Here's the drawing with two shaded views (mm, measured from the low corner). I have some questions. A direction names the side the tool comes from. Give positions to 0.01 mm unless a question says otherwise; leave off trailing zeros. Loops run counter-clockwise (first coordinate to the right, second up) from the corner with the lowest first, then second, coordinate; pieces in that order, holes last. Notation, with made-up numbers: (-11, -12) - (44, -12) arc R35 cw to (44, 23) - close; hole circle Ø3 at (57, 86). An arc over 180 degrees is marked (long way). Write each question's results on one line, items separated by ' | '. Start each with the question number.
1) I want a section at C-C, the plane z = 9. Write out the boundary of the cut face in (x, y).
2) I want a section at A-A, the plane y = 30. Write out the boundary of the cut face in (x, z), and give its area (3 significant figures).
3) I want a section at B-B, the plane x = 22.5. Write out the boundary of the cut face in (y, z), and give its area (3 significant figures).
4) I'm going to push flat-ended pins straight in: pin 1 (3 mm diameter, centred on x = 10.5, z = 27.5, fed in from +Y); pin 2 (10 mm diameter, centred on y = 20, z = 8, fed in from +X); pin 3 (3 mm diameter, centred on x = 9, y = 8, fed in from -Z). Where does each tip first touch, or does it pass through?
5) On a 3-axis mill with a long thin cutter (end or side, diameter ignored), from which of +Z, -Z, +X, -X, +Y, -Y can I reach the whole of each face in a straight line? I mean the marked faces 1 and 2. Say none if no direction works.
6) If I drill on probe 1 along Z at (x, y) = (14.5, 4); probe 2 along Y at (x, z) = (22, 28.5); probe 3 along Z at (x, y) = (16.5, 28.5), over which ranges is the centre line in solid material (lowest first)? Write a range as [from, to].
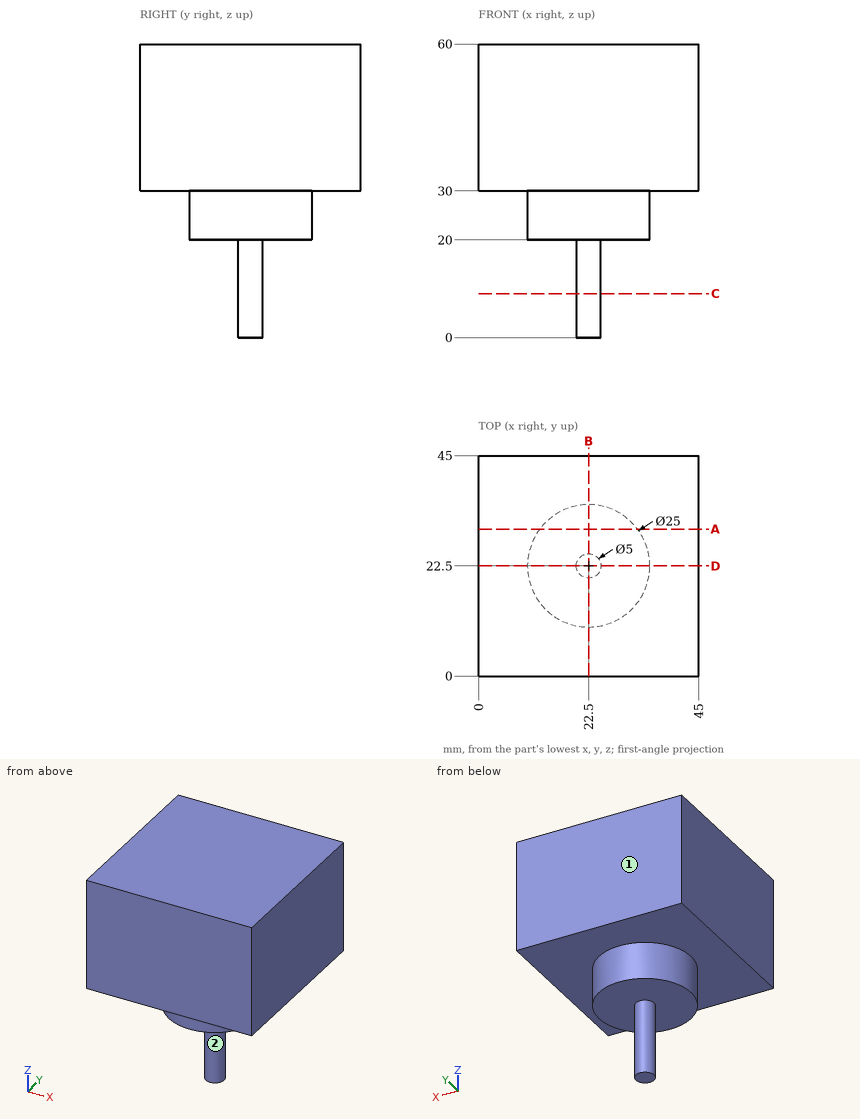
Answers:
1) outline: circle Ø5 at (22.5, 22.5)
2) outline: (0, 30) - (12.5, 30) - (12.5, 20) - (32.5, 20) - (32.5, 30) - (45, 30) - (45, 60) - (0, 60) - close | area: 1,550 mm2
3) outline: (0, 30) - (10, 30) - (10, 20) - (20, 20) - (20, 0) - (25, 0) - (25, 20) - (35, 20) - (35, 30) - (45, 30) - (45, 60) - (0, 60) - close | area: 1,700 mm2
4) pin 1: stops at y = 29.28 | pin 2: stops at x = 25 | pin 3: stops at z = 30
5) face 1: +Z, -Z, +X, -X, +Y | face 2: -Z
6) probe 1: z = [30, 60] | probe 2: y = [10.01, 34.99] | probe 3: z = [20, 60]
